from build123d import *

# Parameters (mm, degrees)
BOX003_W          = 5
BOX003_H          = 22
BOX003_DEPTH      = 2
BOX_W             = 5
BOX_H             = 22
BOX_DEPTH         = 2
CYLINDER006_R     = 2.95
CYLINDER006_DEPTH = 25
CYLINDER007_R     = 2.85
CYLINDER007_DEPTH = 25
BOX002_W          = 62
BOX002_H          = 8
BOX002_DEPTH      = 22
CYLINDER010_R     = 2
CYLINDER010_DEPTH = 10
BOX004_W          = 6.5
BOX004_H          = 3.5
BOX004_DEPTH      = 6.5
PRISM002_DEPTH    = 3.5
CYLINDER009_R     = 2.85
CYLINDER009_DEPTH = 25
CYLINDER008_R     = 10
CYLINDER008_DEPTH = 13
CYLINDER011_R     = 10.95
CYLINDER011_DEPTH = 13


with BuildPart() as cubo003:
    # Box003 → Box003 (new body)
    with BuildSketch(Plane(origin=(28, -11, 6), x_dir=(1, 0, 0), z_dir=(0, 0, 1))):
        with Locations((2.5, 11)):
            Rectangle(BOX003_W, BOX003_H)
    extrude(amount=BOX003_DEPTH)


with BuildPart() as cubo:
    # Box → Box (new body)
    with BuildSketch(Plane(origin=(-33, -11, 6), x_dir=(1, 0, 0), z_dir=(0, 0, 1))):
        with Locations((2.5, 11)):
            Rectangle(BOX_W, BOX_H)
    extrude(amount=BOX_DEPTH)


with BuildPart() as cilindro006:
    # Cylinder006 → Cylinder006 (new body)
    with BuildSketch(Plane.XY.offset(-7)):
        Circle(CYLINDER006_R)
    extrude(amount=CYLINDER006_DEPTH)


with BuildPart() as cilindro007:
    # Cylinder007 → Cylinder007 (new body)
    with BuildSketch(Plane.XY.offset(-7)):
        Circle(CYLINDER007_R)
    extrude(amount=CYLINDER007_DEPTH)


with BuildPart() as cut:
    # Box002 → Box002 (new body)
    with BuildSketch(Plane(origin=(-31, 11, 0), x_dir=(1, 0, 0), z_dir=(0, -1, 0))):
        with Locations((31, 4)):
            Rectangle(BOX002_W, BOX002_H)
    extrude(amount=BOX002_DEPTH)

    # Cut: cut Cilindro007
    add(cilindro007.part, mode=Mode.SUBTRACT)


with BuildPart() as cilindro010:
    # Cylinder010 → Cylinder010 (new body)
    with BuildSketch(Plane(origin=(0, 11, 9), x_dir=(1, 0, 0), z_dir=(0, -1, 0))):
        Circle(CYLINDER010_R)
    extrude(amount=CYLINDER010_DEPTH)


with BuildPart() as cubo004:
    # Box004 → Box004 (new body)
    with BuildSketch(Plane(origin=(-3.25, 4.75, 9), x_dir=(1, 0, 0), z_dir=(0, 0, 1))):
        with Locations((3.25, 1.75)):
            Rectangle(BOX004_W, BOX004_H)
    extrude(amount=BOX004_DEPTH)


with BuildPart() as prisma002:
    # Prism002 → Prism002 (new body)
    with BuildSketch(Plane(origin=(0, 8, 9), x_dir=(1, 0, 0), z_dir=(0, -1, 0))):
        Polygon((3.5, 0), (1.75, 3.031089), (-1.75, 3.031089), (-3.5, 0), (-1.75, -3.031089), (1.75, -3.031089), align=None)
    extrude(amount=PRISM002_DEPTH)


with BuildPart() as cilindro009:
    # Cylinder009 → Cylinder009 (new body)
    with BuildSketch(Plane.XY.offset(-7)):
        Circle(CYLINDER009_R)
    extrude(amount=CYLINDER009_DEPTH)


with BuildPart() as fusion004:
    # Cylinder008 → Cylinder008 (new body)
    with BuildSketch(Plane.XY):
        Circle(CYLINDER008_R)
    extrude(amount=CYLINDER008_DEPTH)

    # Cut007: cut Cilindro009
    add(cilindro009.part, mode=Mode.SUBTRACT)

    # Cut008: cut Prisma002
    add(prisma002.part, mode=Mode.SUBTRACT)

    # Cut009: cut Cubo004
    add(cubo004.part, mode=Mode.SUBTRACT)

    # Cut010: cut Cilindro010
    add(cilindro010.part, mode=Mode.SUBTRACT)


with BuildPart() as fusion004_1:
    # Cut010 placement: moved
    add(fusion004.part.moved(Location((0, 0, 3))))

    # Fusion002: union Cut
    add(cut.part)

    # Cut011: cut Cilindro006
    add(cilindro006.part, mode=Mode.SUBTRACT)

    # Fusion003: union Cubo
    add(cubo.part)

    # Fusion004: union Cubo003
    add(cubo003.part)


with BuildPart() as fusion004003:
    # Cylinder011 → Cylinder011 (new body)
    with BuildSketch(Plane.XY.offset(-10)):
        Circle(CYLINDER011_R)
    extrude(amount=CYLINDER011_DEPTH)

    # Fusion004003: union Fusion004
    add(fusion004_1.part)


solid = fusion004003.part
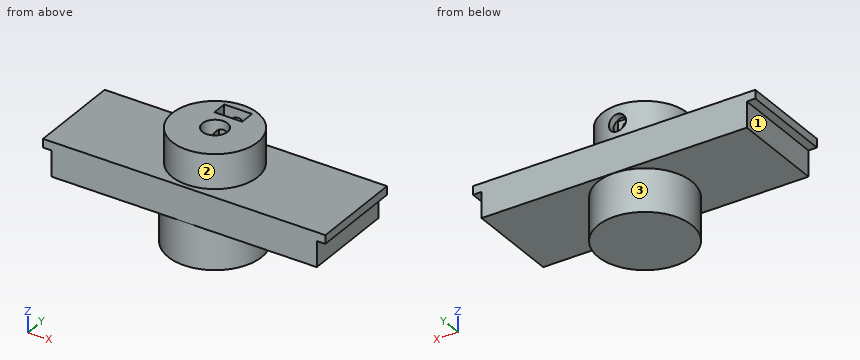
Can you work these out from the model? Positions are in its coordinate system, mm. Face numbers are marked on the shaded views. A direction names the side the tool comes from. Give positions to 0.01 mm unless a question says otherwise; leave off trailing zeros. Loops run counter-clockwise (first coordinate to the right, second up) from the corner with the lowest first, then second, coordinate; pieces in that order, holes last. Notation, with made-up numbers: (7, 1) - (26, 1) arc R14 ccw to (26, 11) - close; hole circle Ø5 at (11.5, 11.25). An arc over 180 degrees is marked (long way). Answer as a JSON object with one key per item and string values.
Q1. Will these pins go through, and if not, where does the flat tip stop? P1, Ø5, axis at y = 4, z = 1.5, coming from the +X side; P2, Ø1.5, axis at x = -1, z = 13, coming from the -Y side; P3, Ø3, axis at x = 0.5, z = 12.5, coming from the +Y side; P4, Ø6.5, axis at x = 0, y = -0.5, coming from the +Z side.
Geometry says:
{"P1": "x = 31", "P2": "y = -10", "P3": "y = 10", "P4": "z = 16"}
Q2. Imagine slicing it at B-B on y = 0. Write out the boundary of the cut face in (x, z).
Geometry says:
{"outline": "(-33, 6) - (-31, 6) - (-31, 0) - (-10.95, 0) - (-10.95, -10) - (10.95, -10) - (10.95, 0) - (31, 0) - (31, 6) - (33, 6) - (33, 8) - (10, 8) - (10, 16) - (2.95, 16) - (2.95, 3) - (-2.95, 3) - (-2.95, 16) - (-10, 16) - (-10, 8) - (-33, 8) - close"}
Q3. Which directions (+Z, -Z, +X, -X, +Y, -Y) give clear straight access to the entire face, cutting with the end or side of a thin tool? Please do the marked faces 1, 2 and 3.
Geometry says:
{"face 1": "-Z, -X, +Y, -Y", "face 2": "+Z", "face 3": "-Z"}
Q4. If I drill on L1, parallel to X at y = 0, z = 12.25; L2, parallel to Y at x = 1.5, z = 13.5; L3, parallel to Z at x = 0, y = 4.05, over which ranges is the centre line in solid material (lowest first)?
Geometry says:
{"L1": "-10 to -2.95, 2.95 to 10", "L2": "-9.89 to -2.54, 2.54 to 4.5, 8.25 to 9.89", "L3": "-10 to 10, 14 to 16"}
Q5. Imagine slicing it at C-C on z = 4.5. Write out the boundary of the cut face in (x, y), plus the area to 3 significant figures.
Geometry says:
{"outline": "(-31, -11) - (31, -11) - (31, 11) - (-31, 11) - close; hole circle Ø5.9 at (0, 0)", "area": "1,340 mm²"}
Q6. Imagine slicing it at D-D on x = -25.5. Write out the boundary of the cut face in (y, z).
Geometry says:
{"outline": "(-11, 0) - (11, 0) - (11, 8) - (-11, 8) - close"}
Q7. Imagine slicing it at A-A on x = 0. Give the number of separate pieces and of enclosed holes in the cut face, plus the area to 3 significant figures.
Geometry says:
{"separate pieces": "3", "enclosed holes": "0", "area": "439 mm²"}
